from build123d import *

# Parameters (mm, degrees)
SKETCH1_W           = 3
SKETCH1_H           = 10
SKETCH1_W_2         = 10
SKETCH1_H_2         = 3
BOSS_EXTRUDE2_DEPTH = 3
FILLET1_R           = 3
SKETCH2_R           = 1.6
CUT_EXTRUDE1_DEPTH  = 3
SKETCH3_R           = 1.5
CUT_EXTRUDE2_DEPTH  = 10
SKETCH4_W           = 20
SKETCH4_H           = 10
CUT_EXTRUDE3_DEPTH  = 10


with BuildPart() as part:
    # Sketch1 → Boss-Extrude2 (new body)
    with BuildSketch(Plane(origin=(0, 0, 0), x_dir=(1, 0, 0), z_dir=(0, 1, 0))):
        Polygon((0, 49.5), (0, 0), (40.5, 0), (50.5, 0), (53.5, 0), (53.5, 3), (52, 3), (52, 6), (53.5, 6), (53.5, 15), (56.5, 15), (56.5, 6), (58, 6), (58, 3), (56.5, 3), (56.5, 0), (59.5, 0), (69.5, 0), (110, 0), (110, 49.5), (110, 59.5), (110, 62.5), (107, 62.5), (107, 61), (104, 61), (104, 62.5), (95, 62.5), (95, 65.5), (104, 65.5), (104, 67), (107, 67), (107, 65.5), (110, 65.5), (110, 68.5), (110, 78.5), (110, 128), (69.5, 128), (59.5, 128), (56.5, 128), (56.5, 125), (58, 125), (58, 122), (56.5, 122), (56.5, 113), (53.5, 113), (53.5, 122), (52, 122), (52, 125), (53.5, 125), (53.5, 128), (50.5, 128), (40.5, 128), (0, 128), (0, 78.5), (0, 68.5), (0, 65.5), (3, 65.5), (3, 67), (6, 67), (6, 65.5), (15, 65.5), (15, 62.5), (6, 62.5), (6, 61), (3, 61), (3, 62.5), (0, 62.5), (0, 59.5), align=None)
        with Locations((111.5, 73.5)):
            Rectangle(SKETCH1_W, SKETCH1_H)
        with Locations((-1.5, 54.5)):
            Rectangle(SKETCH1_W, SKETCH1_H)
        with Locations((-1.5, 73.5)):
            Rectangle(SKETCH1_W, SKETCH1_H)
        with Locations((45.5, -1.5)):
            Rectangle(SKETCH1_W_2, SKETCH1_H_2)
        with Locations((45.5, 129.5)):
            Rectangle(SKETCH1_W_2, SKETCH1_H_2)
        with Locations((64.5, 129.5)):
            Rectangle(SKETCH1_W_2, SKETCH1_H_2)
        with Locations((64.5, -1.5)):
            Rectangle(SKETCH1_W_2, SKETCH1_H_2)
        with Locations((111.5, 54.5)):
            Rectangle(SKETCH1_W, SKETCH1_H)
    extrude(amount=BOSS_EXTRUDE2_DEPTH)

    # Fillet1
    fillet1_edges = [part.edges().sort_by_distance(p)[0] for p in [
        (0, 1.5, 0),
        (0, 1.5, -128),
        (110, 1.5, -128),
        (110, 1.5, 0),
    ]]
    fillet(fillet1_edges, radius=FILLET1_R)

    # Sketch2 → Cut-Extrude1 (cut)
    with BuildSketch(Plane(origin=(0, 3, 0), x_dir=(1, 0, 0), z_dir=(0, 1, 0))):
        with Locations(Location((74.05, 81.5, 0), (0, 0, 270))):
            Circle(SKETCH2_R)
        with Locations(Location((46.11, 81.5, 0), (0, 0, 270))):
            Circle(SKETCH2_R)
        with Locations(Location((79.15, 29.4, 0), (0, 0, 270))):
            Circle(SKETCH2_R)
        with Locations(Location((30.91, 30.7, 0), (0, 0, 270))):
            Circle(SKETCH2_R)
    extrude(amount=-CUT_EXTRUDE1_DEPTH, mode=Mode.SUBTRACT)

    # Sketch3 → Cut-Extrude2 (cut)
    with BuildSketch(Plane(origin=(0, 3, 0), x_dir=(1, 0, 0), z_dir=(0, 1, 0))):
        with Locations(Location((98, 6, 0), (0, 0, 270))):
            Circle(SKETCH3_R)
        with Locations(Location((104, 6, 0), (0, 0, 270))):
            Circle(SKETCH3_R)
    extrude(amount=-CUT_EXTRUDE2_DEPTH, mode=Mode.SUBTRACT)

    # Sketch4 → Cut-Extrude3 (cut)
    with BuildSketch(Plane(origin=(0, 3, 0), x_dir=(1, 0, 0), z_dir=(0, 1, 0))):
        with Locations((13, 120)):
            Rectangle(SKETCH4_W, SKETCH4_H)
    extrude(amount=-CUT_EXTRUDE3_DEPTH, mode=Mode.SUBTRACT)


solid = part.part
Input: part model. Units: mm. Frame: model coordinates. A direction names the side the tool comes from. Coordinates: 2 decimals unless noted, no trailing zeros. Loops run counter-clockwise (first coordinate to the right, second up) from the corner with the lowest first, then second, coordinate; pieces in that order, holes last.
(1) First-contact query: pin 1 Ø1.5 at (x, y) = (108.5, 1.5) entering from +Z; pin 2 Ø1.5 at (x, y) = (1.5, 2) entering from -Z; pin 3 Ø3 at (x, z) = (30.91, -30.7) entering from +Y. Flat tips, straight axial feed; report the tip coordinate or a pass-through.
(2) Section A-A on x = 98. Return the cut outline in (y, z).
(3) Pull-direction query (X, two-part tool) for faces 1 (the face through (45, 1, 3)), 2 (the face through (31.391, 1.521, -29.174)), 3 (the face through (69.5, 1, 2)); classes: released by +X, released by -X, zero draft, split by the parting line, or undercut.
(4) Section C-C on x = 30.91. Return the cut outline in (y, z), then the cut area to 3 significant figures.
(5) Set-up query: faces 4 (the face through (59.5, 1, 2)), 5 (the face through (106, 1, -61)), 6 (the face through (1, 1, -65.5)), 7 (the face through (110, 1, -67)), 8 (the face through (111, 1, -78.5)). Return all of +Z, -Z, +X, -X, +Y, -Y with unobstructed straight access to the full face (end or side cutting, diameter ignored); none if empty.
(6) Section D-D on z = -48. Return the cut outline in (x, y), then the cut area to 3 significant figures.
(7) Section B-B on x = 46.11. Return the cut outline in (y, z).
(8) Material intervals for probe 1 along X at (y, z) = (1.9, -116); probe 2 along X at (y, z) = (1.55, -81.5); probe 3 along Z at (x, y) = (98, 1.35), sorted ascending.
Data:
1. pin 1: stops at z = -0.1
1. pin 2: stops at z = -127.9
1. pin 3: passes through
2. outline: (0, -128) - (3, -128) - (3, -65.5) - (0, -65.5) - close; (0, -62.5) - (3, -62.5) - (3, -7.5) - (0, -7.5) - close; (0, -4.5) - (3, -4.5) - (3, 0) - (0, 0) - close
3. face 1: zero draft
3. face 2: undercut
3. face 3: released by +X
4. outline: (0, -128) - (3, -128) - (3, -32.3) - (0, -32.3) - close; (0, -29.1) - (3, -29.1) - (3, 0) - (0, 0) - close
4. area: 374 mm2
5. face 4: +Z, +Y, -Y
5. face 5: +Y, -Y
5. face 6: -X, +Y, -Y
5. face 7: +X, +Y, -Y
5. face 8: -Z, +X, +Y, -Y
6. outline: (0, 0) - (110, 0) - (110, 3) - (0, 3) - close
6. area: 330 mm2
7. outline: (0, -131) - (3, -131) - (3, -83.1) - (0, -83.1) - close; (0, -79.9) - (3, -79.9) - (3, 3) - (0, 3) - close
8. probe 1: x = 0 to 3, 23 to 53.5, 56.5 to 110
8. probe 2: x = 0 to 44.51, 47.71 to 72.45, 75.65 to 110
8. probe 3: z = -128 to -65.5, -62.5 to -7.5, -4.5 to 0
